Input: part model. Units: mm. Frame: model coordinates. A direction names the side the tool comes from. Coordinates: 2 decimals unless noted, no trailing zeros. Loops run counter-clockwise (first coordinate to the right, second up) from the corner with the lowest first, then second, coordinate; pieces in that order, holes last. Notation, with made-up numbers: (-17.5, -12.5) -> (22.5, -12.5) arc R32 cw to (22.5, 20.5) -> close; hole circle Ø3 at (-40, -1.75). An arc over 180 degrees is marked (long way). Put each result on its own line as item: value. Start each with the question number.
1) Set-up query: faces 4 (the flat face through (0, 0, 0)), 5 (the flat face through (-1.42, 30, 3.92)). Return all of +Z, -Z, +X, -X, +Y, -Y with unobstructed straight access to the full face (end or side cutting, diameter ignored); none if empty.
2) Cut plane B-B (x = 0). Return the cut outline in (y, z), plus the area to 3 significant figures.
3) Pull-direction query (Z, two-part tool) for faces 1 (the flat face through (1, 33, -3)), 2 (the cylindrical face through (-3, 32, 0)), 3 (the cylindrical face through (-6, 15, 0)); classes: pulls with the +Z half, pulls with the -Z half, needs draft (parallel to the pull), parting line crosses it, or undercut.
4) Cut plane D-D (z = -3.5). Return the cut outline in (x, y), plus the area to 3 significant figures.
5) Cut plane A-A (z = 0). Return the cut outline in (x, y).
6) Contact query for flat-ended pins moving along their axis: P1, Ø2, axis at x = -2.5, y = 9.5, coming from the +Z side; P2, Ø5, axis at x = 0, z = 0, coming from the +Y side; P3, Ø5, axis at x = -3.5, y = 25.5, coming from the -Z side. Output: stop coordinate, or through.
7) Cut plane C-C (y = 18). Return the cut outline in (x, z).
8) Material intervals for L1, parallel to X at y = 30.7, z = 0; L2, parallel to Y at x = 5.25, z = -2.75, sorted ascending.
from build123d import *

# Parameters (mm, degrees)
SKETCH2_R           = 6
BOSS_EXTRUDE1_DEPTH = 30
SKETCH3_R           = 4
BOSS_EXTRUDE2_DEPTH = 3
SKETCH4_R           = 3
CUT_EXTRUDE1_DEPTH  = 3


with BuildPart() as part:
    # Sketch2 → Boss-Extrude1 (new body)
    with BuildSketch(Plane(origin=(0, 0, 0), x_dir=(1, 0, 0), z_dir=(0, 1, 0))):
        Circle(SKETCH2_R)
    extrude(amount=BOSS_EXTRUDE1_DEPTH)

    # Sketch3 → Boss-Extrude2 (add)
    with BuildSketch(Plane(origin=(0, 30, 0), x_dir=(1, 0, 0), z_dir=(0, 1, 0))):
        Circle(SKETCH3_R)
    extrude(amount=BOSS_EXTRUDE2_DEPTH)

    # Sketch4 → Cut-Extrude1 (cut)
    with BuildSketch(Plane(origin=(0, 33, 0), x_dir=(1, 0, 0), z_dir=(0, 1, 0))):
        Circle(SKETCH4_R)
    extrude(amount=-CUT_EXTRUDE1_DEPTH, mode=Mode.SUBTRACT)


solid = part.part
Results found:
1. face 4: +Z, -Z, +X, -X, -Y
1. face 5: +Y
2. outline: (0, -6) -> (30, -6) -> (30, -4) -> (33, -4) -> (33, -3) -> (30, -3) -> (30, 3) -> (33, 3) -> (33, 4) -> (30, 4) -> (30, 6) -> (0, 6) -> close
2. area: 366 mm2
3. face 1: needs draft
3. face 2: undercut
3. face 3: parting line crosses it
4. outline: (-4.87, 0) -> (4.87, 0) -> (4.87, 30) -> (1.94, 30) -> (1.94, 33) -> (-1.94, 33) -> (-1.94, 30) -> (-4.87, 30) -> close
4. area: 304 mm2
5. outline: (-6, 0) -> (6, 0) -> (6, 30) -> (4, 30) -> (4, 33) -> (3, 33) -> (3, 30) -> (-3, 30) -> (-3, 33) -> (-4, 33) -> (-4, 30) -> (-6, 30) -> close
6. P1: stops at z = 5.81
6. P2: stops at y = 30
6. P3: stops at z = -5.92
7. outline: circle Ø12 at (0, 0)
8. L1: x = -4 to -3, 3 to 4
8. L2: y = 0 to 30
